Autodesk Fusion 360 part; units mm, degrees
sketch "Sketch1" plane through (0, 0, 0) normal (0, 0, 1) x (1, 0, 0)
  line L0 (0, 0) -> (15.8, 0)
  line L1 (15.8, 0) -> (15.8, 15.8)
  line L2 (15.8, 15.8) -> (0, 15.8)
  line L3 (0, 15.8) -> (0, 0)
  circle A0 centre (3.9, 11.9) radius 2.4
  circle A1 centre (11.9, 11.9) radius 2.4
  circle A2 centre (11.9, 3.9) radius 2.4
  circle A3 centre (3.9, 3.9) radius 2.4
  line L4 (1.2, 1.2) -> (14.6, 1.2)
  line L5 (14.6, 1.2) -> (14.6, 14.6)
  line L6 (14.6, 14.6) -> (1.2, 14.6)
  line L7 (1.2, 14.6) -> (1.2, 1.2)
  circle A4 centre (7.9, 7.9) radius 3.255
  circle A5 centre (7.9, 7.9) radius 2.4
  circle A6 centre (3.9, 11.9) radius 1.3
  circle A7 centre (11.9, 11.9) radius 1.3
  circle A8 centre (11.9, 3.9) radius 1.3
  circle A9 centre (3.9, 3.9) radius 1.3
  dimension "d1" = 15.8
  dimension "d2" = 15.8
  dimension "d3" = 4.8
  dimension "d4" = 4.8
  dimension "d5" = 4.8
  dimension "d6" = 4.8
  dimension "d7" = 8
  dimension "d8" = 8
  dimension "d9" = 8
  dimension "d10" = 8
  dimension "d11" = 3.9
  dimension "d12" = 3.9
  dimension "d13" = 3.9
  dimension "d14" = 13.4
  dimension "d15" = 13.4
  dimension "d16" = 1.2
  dimension "d17" = 1.2
  dimension "d18" = 6.51
  dimension "d19" = 6.7
  dimension "d20" = 6.7
  dimension "d21" = 4.8
  dimension "d22" = 2.6
  dimension "d23" = 2.6
  dimension "d24" = 2.6
  dimension "d25" = 2.6
  dimension "d32" = 3.9
extrude "Extrude1" add sketch "Sketch1" along normal blind 9.6 contours L0 L1 L2 L3 | A4 makes body 1 at (0, 10.5333, 3.2) makes body 2 at (11.1388, 8.2241, 6.4)
extrude "Extrude2" add sketch "Sketch1" along normal blind 9.6 and the other way blind -8.6 contours A0 | A1 | A2 | A3 | L4 L5 L6 L7 | A5 bodies 1 2
extrude "Extrude3" add sketch "Sketch1" along normal blind 11.4 and the other way blind -9.6 contours A0 | A1 | A2 | A3 | A6 | A7 | A8 | A9 bodies 1
extrude "Extrude4" cut sketch "Sketch1" along normal blind 10.3 contours A6 | A7 | A8 | A9 bodies 1
copy_body "Body->Comp1" bodies 1 removing the originals makes body 3 in component "Yellow 2x2"
component "Yellow 2x2" placed x (1, 0, 0) y (0, 1, 0) z (0, 0, 1) at (0, 0, 0)
equation "d14 = 15.8 mm - 1.2 mm - 1.2 mm"
equation "d15 = 15.8 mm - 1.2 mm - 1.2 mm"
equation "d19 = ( 13.4 / 2 ) * 1 mm"
equation "d33 = 9.6 mm + 1.8 mm"
equation "d37 = 9.6 mm + 0.7 mm"
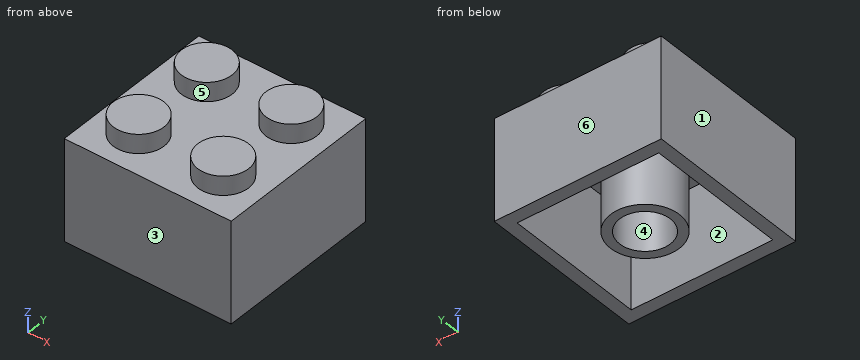
Input: part model. Units: mm. Frame: model coordinates. Face numbers are marked on the shaded views. A direction names the side the tool comes from. Round coordinates to 2 decimals unless told otherwise and drop trailing zeros. Loops run counter-clockwise (first coordinate to the right, second up) from the corner with the lowest first, then second, coordinate; pieces in that order, holes last.
1) Section query B-B on y = 7.9. Return the cut outline in (x, z) (3 decimals), plus the area to 3 significant figures.
Ans:
outline: (0, 0) - (1.2, 0) - (1.2, 8.6) - (4.645, 8.6) - (4.645, 0) - (5.5, 0) - (5.5, 8.6) - (10.3, 8.6) - (10.3, 0) - (11.155, 0) - (11.155, 8.6) - (14.6, 8.6) - (14.6, 0) - (15.8, 0) - (15.8, 9.6) - (0, 9.6) - close
area: 51.1 mm2
2) Set-up query: the marked faces 4, 5 and 6. Return all of +Z, -Z, +X, -X, +Y, -Y with unobstructed straight access to the full face (end or side cutting, diameter ignored); none if empty.
Ans:
face 4: -Z
face 5: +Z
face 6: +Z, -Z, +X, -X, +Y
3) Pin query (flat end, axial travel): pin 1 (2.5 mm diameter, centred on x = 7.5, y = 7, fed in from -Z); pin 2 (0.8 mm diameter, centred on x = 4, y = 3.5, fed in from -Z); pin 3 (5.5 mm diameter, centred on x = 7.9, y = 7.9, fed in from +Z). Return the tip coordinate at first contact, or that it passes through.
Ans:
pin 1: stops at z = 8.6
pin 2: stops at z = 10.3
pin 3: stops at z = 9.6
4) Pull-direction query (Y, two-part tool) for the marked faces 1, 2 and 3; classes: released by +Y, released by -Y, zero draft, split by the parting line, or undercut.
Ans:
face 1: zero draft
face 2: undercut
face 3: released by -Y
5) Material intervals for line 1 (Y direction, x = 11.9, z = 9.2); line 2 (Y direction, x = 11.9, z = 9.65); line 3 (X direction, y = 12.25, z = 0.5), sorted ascending.
Ans:
line 1: y = 0 to 2.6, 5.2 to 10.6, 13.2 to 15.8
line 2: y = 1.5 to 2.6, 5.2 to 6.3, 9.5 to 10.6, 13.2 to 14.3
line 3: x = 0 to 1.2, 14.6 to 15.8
6) Section query D-D on y = 3.9. Return the cut outline in (x, z), plus the area to 3 significant figures.
Ans:
outline: (0, 0) - (1.2, 0) - (1.2, 8.6) - (2.6, 8.6) - (2.6, 10.3) - (5.2, 10.3) - (5.2, 8.6) - (10.6, 8.6) - (10.6, 10.3) - (13.2, 10.3) - (13.2, 8.6) - (14.6, 8.6) - (14.6, 0) - (15.8, 0) - (15.8, 9.6) - (14.3, 9.6) - (14.3, 11.4) - (9.5, 11.4) - (9.5, 9.6) - (6.3, 9.6) - (6.3, 11.4) - (1.5, 11.4) - (1.5, 9.6) - (0, 9.6) - close
area: 44.9 mm2
7) Section query A-A on z = 1.5. Return the cut outline in (x, y) (3 decimals), plus the area to 3 significant figures.
Ans:
outline: (0, 0) - (15.8, 0) - (15.8, 15.8) - (0, 15.8) - close; circle Ø6.51 at (7.9, 7.9); hole (1.2, 1.2) - (14.6, 1.2) - (14.6, 14.6) - (1.2, 14.6) - close; hole circle Ø4.8 at (7.9, 7.9)
area: 85.3 mm2
